Can you work these out from the model? Positions are in its coordinate system, mm. A direction names the side the tool comes from. Give positions to 0.01 mm unless a question says otherwise; leave off trailing zeros. Use CSV: the item, a comma, the result in double quotes. Start each with the question number.
from build123d import *

# Parameters (mm, degrees)
CUT_EXTRUDE_START        = 16.5
CUT_EXTRUDE_1_DEPTH      = 14
PATTERN_CIRCULAR_1_COUNT = 14
SKETCH_6_R               = 4
CUT_EXTRUDE_2_DEPTH      = 28.440845468
CHAMFER_1_SIZE           = 0.18
SKETCH_10_W              = 3
SKETCH_10_H              = 6.5


with BuildPart() as part:
    # 草图3 → 旋转1 (revolve)
    with BuildSketch(Plane.XY):
        Polygon((0, 0), (0, 8.475), (0.275, 8.75), (2.5, 8.75), (2.5, 11.065), (16.5, 11.065), (16.5, 8.75), (18.725, 8.75), (19, 8.475), (19, 0), align=None)
    revolve(axis=Axis((19, 0, 0), (-1, 0, 0)))

    # 草图4 → Cut-Extrude 1 (cut)
    with BuildSketch(Plane(origin=(0, 0, 0), x_dir=(0, 0, -1), z_dir=(1, 0, 0)).offset(CUT_EXTRUDE_START)):
        with BuildLine():
            Line((-0.246387141, 9.665), (0.246387141, 9.665))
            ThreePointArc((0.246387141, 9.665), (0.574139902, 9.760531218), (0.799234891, 10.01720286))
            Line((0.799234891, 10.01720286), (1.064880338, 10.58688136))
            ThreePointArc((1.064880338, 10.58688136), (1.330886548, 10.867435343), (1.712114902, 10.931737628))
            ThreePointArc((1.712114902, 10.931737628), (0, 11.065), (-1.712114902, 10.931737628))
            ThreePointArc((-1.712114902, 10.931737628), (-1.330886548, 10.867435343), (-1.064880338, 10.58688136))
            Line((-1.064880338, 10.58688136), (-0.799234891, 10.01720286))
            ThreePointArc((-0.799234891, 10.01720286), (-0.574139902, 9.760531218), (-0.246387141, 9.665))
        make_face()
    cut_extrude_1 = extrude(amount=-CUT_EXTRUDE_1_DEPTH, mode=Mode.SUBTRACT)

    # 阵列(圆周)1: Cut-Extrude 1 ×14 about axis
    pattern_circular_1_axis = Axis((0, 0, 0), (1, 0, 0))
    for i in range(1, PATTERN_CIRCULAR_1_COUNT):
        add(cut_extrude_1.rotate(pattern_circular_1_axis, i * 360 / PATTERN_CIRCULAR_1_COUNT), mode=Mode.SUBTRACT)

    # 草图5 → 旋转2 (revolve)
    with BuildSketch(Plane.XY, mode=Mode.PRIVATE) as revolve_2_sk:
        Polygon((1.95, 14), (2.5, 11.065), (2.5, 8.75), (1.5, 8.75), (1.5, 11.065), (0.95, 14), align=None)
        Polygon((17.5, 8.75), (16.5, 8.75), (16.5, 11.065), (17.05, 14), (18.05, 14), (17.5, 11.065), align=None)
    revolve(revolve_2_sk.sketch.rotate(Axis((0, 0, 0), (1, 0, 0)), 180), axis=Axis((0, 0, 0), (1, 0, 0)))

    # 草图6 → 切除-拉伸2 (cut, through all)
    with BuildSketch(Plane(origin=(0, 0, 0), x_dir=(0, 0, -1), z_dir=(1, 0, 0))):
        Circle(SKETCH_6_R)
    extrude(amount=CUT_EXTRUDE_2_DEPTH, mode=Mode.SUBTRACT)

    # 倒角1
    chamfer_1_edges = [part.edges().sort_by_distance(p)[0] for p in [
        (0, 0, 4),
        (19, 0, 4),
    ]]
    chamfer(chamfer_1_edges, length=CHAMFER_1_SIZE)

    # 草图10 → Cut-Revolve 8317 (revolve, cut)
    with BuildSketch(Plane.XY, mode=Mode.PRIVATE) as cut_revolve_8317_sk:
        with Locations((17.5, 3.25)):
            Rectangle(SKETCH_10_W, SKETCH_10_H)
        with Locations((1.5, 3.25)):
            Rectangle(SKETCH_10_W, SKETCH_10_H)
    revolve(cut_revolve_8317_sk.sketch.rotate(Axis((0, 0, 0), (1, 0, 0)), 90), axis=Axis((0, 0, 0), (1, 0, 0)), mode=Mode.SUBTRACT)


solid = part.part
(1) Thinking about a two-plate mould opening in Y: for faces 4 (the face through (9.6, 8.64, 6.91)), 5 (the face through (16.5, 10.5, 0)), 6 (the face through (16.5, -7, 8)), 7 (the face through (16.5, 6, -8)), which applies, released by +Y, released by -Y, zero draft, split by the parting line, or undercut?
(2) Will these pins go through, and if not, where does the flat tip stop? pin 1 Ø8 at (x, y) = (17, -8.5) entering from +Z; pin 2 Ø3 at (x, z) = (9.5, -2) entering from +Y; pin 3 Ø15 at (y, z) = (0, 0) entering from +X; pin 4 Ø1 at (y, z) = (9, 5) entering from -X.
(3) Please list where these lines run through material, in increasing order: L1, parallel to Z at x = 8.5, y = 0.25; L2, parallel to Y at x = 8.5, z = 0 (3 decimals); L3, parallel to Y at x = 0.8, z = 0. Write a range as [from, to].
(4) Which directions (+Z, -Z, +X, -X, +Y, -Y) give clear straight access to the entire face, cutting with the end or side of a thin tool? Please do faces 1 (the face through (16.5, -2, 10)), 2 (the face through (16.5, -2, -10)), 3 (the face through (9.598, -10.785, -2.473)).
Geometry results:
1,face 4,"released by +Y"
1,face 5,"zero draft"
1,face 6,"undercut"
1,face 7,"undercut"
2,pin 1,"stops at z = 13.26"
2,pin 2,"stops at y = 10.94"
2,pin 3,"stops at x = 19"
2,pin 4,"stops at x = 1.5"
3,L1,"z = [-11.06, -3.99], [3.99, 11.06]"
3,L2,"y = [-9.665, -4], [4, 9.665]"
3,L3,"y = [-8.75, -6.5], [6.5, 8.75]"
4,face 1,"+Z"
4,face 2,"-Z"
4,face 3,"-Z, -Y"
